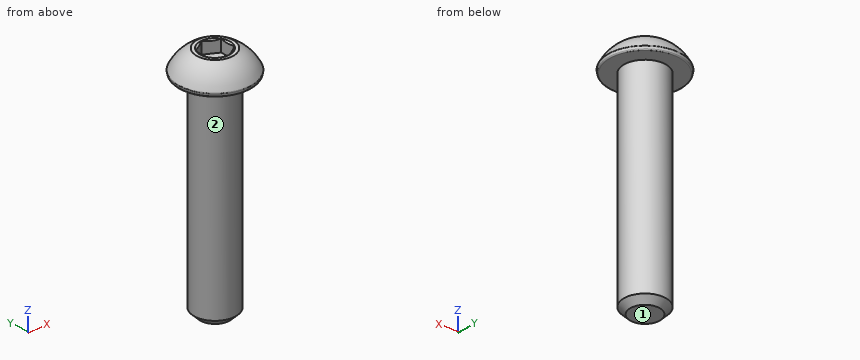
```python
from build123d import *

# Parameters (mm, degrees)
CUT_EXTRUDE1_DEPTH = 1.84404
FILLET1_R          = 0.16764


with BuildPart() as part:
    # Sketch2 → Revolve1 (revolve)
    with BuildSketch(Plane(origin=(0, 0, 0), x_dir=(0, 0, -1), z_dir=(1, 0, 0))):
        with BuildLine():
            Line((31.75, 0), (-3.3528, 0))
            Line((-3.3528, 0), (-3.3528, 2.778125))
            ThreePointArc((-3.3528, 2.778125), (-2.158424687, 4.401074199), (-0.50292, 5.5499))
            Line((-0.50292, 5.5499), (0, 5.461221635))
            Line((0, 5.461221635), (0, 3.175))
            Line((0, 3.175), (30.7975, 3.175))
            Line((30.7975, 3.175), (31.75, 2.2225))
            Line((31.75, 2.2225), (31.75, 0))
        make_face()
    revolve(axis=Axis((0, 0, -31.75), (0, 0, 1)))

    # Sketch3 → Cut-Extrude1 (cut)
    with BuildSketch(Plane.XY.offset(3.3528)):
        Polygon((0, 2.291358881), (-1.984375, 1.14567944), (-1.984375, -1.14567944), (0, -2.291358881), (1.984375, -1.14567944), (1.984375, 1.14567944), align=None)
    extrude(amount=-CUT_EXTRUDE1_DEPTH, mode=Mode.SUBTRACT)

    # Cut-Extrude2 cone 1 section (through the dimple's axis) → Cut-Extrude2 (revolve, cut)
    with BuildSketch(Plane(origin=(0, 0, 3.3528), x_dir=(0, -1, 0), z_dir=(1, 0, 0))):
        Polygon((0, 0), (2.291358881, 0), (0, 1.322916667), align=None)
    revolve(axis=Axis((0, 0, 3.3528), (0, 0, -1)), mode=Mode.SUBTRACT)

    # Fillet1
    fillet1_edges = [part.edges().sort_by_distance(p)[0] for p in [
        (0, -5.5499, 0.50292),
        (0, -5.461221635, 0),
    ]]
    fillet(fillet1_edges, radius=FILLET1_R)


solid = part.part
```
Design review of the part built by this model. Coordinates are the model's own, in mm. Face numbers are marked on the shaded views. A direction names the side the tool comes from. Round coordinates to 2 decimals unless told otherwise and drop trailing zeros. Order: outer loops, then holes, each group sorted by start corner. A loop starts at its lowest first (then second) coordinate and runs counter-clockwise, first axis right, second up. Notation, with made-up numbers: M 32,-13.75 L 38,-13.75 A24 ccw 38,6.25 Z; hole C 68.25,-5.75 d2. An arc over 180 degrees is marked long. Put each result on its own line as item: value.
Q1. To check wall thickness, follow line 1 (Z direction, x = -0.75, y = 1.5); line 2 (Y direction, x = 0, z = -11.5) (3 decimals); line 3 (X direction, y = 0.25, z = -6.5). State the ranges of each line that lie inside material, in increasing order.
Reported:
line 1: -31.75 to 1.51
line 2: -3.175 to 3.175
line 3: -3.17 to 3.17
Q2. Consider section A-A (z = -28.5). State the section outline as (x, y) points (3 decimals), and give its area (3 significant figures).
Reported:
outline: C 0,0 d6.35
area: 31.7 mm²
Q3. Insertion check: pin 1 Ø0.9 at (y, z) = (0, 2.5) entering from -X; pin 2 Ø1.2 at (x, y) = (-0.5, 0) entering from +Z; pin 3 Ø4 at (y, z) = (1, -21) entering from -X (3 decimals). Each pin has a flat end and moves straight along its axis. Give the tip position at first contact, or say it passes through.
Reported:
pin 1: x = -4.5
pin 2: z = 1.51
pin 3: x = -3.175
Q4. Machinability: for the marked faces 1 and 2, which of the approach directions +Z, -Z, +X, -X, +Y, -Y give a long, thin tool a straight path to every point of the face, cutting with its end or side? Answer none if there is none.
Reported:
face 1: -Z, +X, -X, +Y, -Y
face 2: -Z
